Could you check a few things on this model? Use its own coordinates, in mm. Face numbers are marked on the shaded views. A direction names the side the tool comes from. Coordinates: 2 decimals unless noted, no trailing zeros. Loops run counter-clockwise (first coordinate to the right, second up) from the corner with the lowest first, then second, coordinate; pieces in that order, holes last.
1) Imagine slicing it at A-A on x = 0. Please give me the cut outline in (y, z).
2) If I drill on line 1 along Y through (x, z) = (0, 3.5); line 2 along Y through (x, z) = (2.25, 0.5); line 3 along X through (y, z) = (2.5, 4.75), over which ranges is the centre line in solid material (lowest first)?
3) For the marked faces 1 and 2, which set-ups out of +Z, -Z, +X, -X, +Y, -Y let a thin tool reach every point of the face, with its end or its side?
4) Will these pins go through, and if not, where does the flat tip stop? P1, Ø4, axis at y = -1, z = 6, coming from the +X side; P2, Ø3, axis at x = 1, z = 5.5, coming from the +Y side; P3, Ø1.5, axis at y = -2.5, z = -0.5, coming from the -X side.
5) Thinking about a two-plate mould opening in Y: for the marked faces 3, 4 and 5, which applies, released by +Y, released by -Y, zero draft, split by the parting line, or undercut?
6) Imagine slicing it at B-B on z = 6.75. Please give me the cut outline in (x, y), plus the area to 3 significant figures.
```python
from build123d import *

# Parameters (mm, degrees)
SKETCH2_R           = 4
SKETCH2_R_2         = 3.5
BOSS_EXTRUDE1_DEPTH = 8
SKETCH3_R           = 5
BOSS_EXTRUDE2_DEPTH = 2
BOSS_EXTRUDE2_TAPER = 30


with BuildPart() as part:
    # Sketch2 → Boss-Extrude1 (new body)
    with BuildSketch(Plane.XY):
        Circle(SKETCH2_R)
        Circle(SKETCH2_R_2, mode=Mode.SUBTRACT)
    extrude(amount=BOSS_EXTRUDE1_DEPTH)

    # Sketch3 → Boss-Extrude2 (add)
    with BuildSketch(Plane(origin=(0, 0, 0), x_dir=(-1, 0, 0), z_dir=(0, 0, -1))):
        Circle(SKETCH3_R)
    extrude(amount=BOSS_EXTRUDE2_DEPTH, taper=BOSS_EXTRUDE2_TAPER)


solid = part.part
```
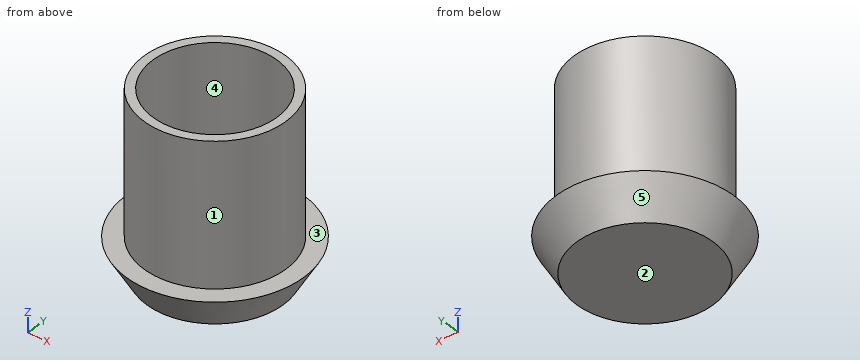
Filled in:
1. outline: (-5, 0) - (-3.85, -2) - (3.85, -2) - (5, 0) - (4, 0) - (4, 8) - (3.5, 8) - (3.5, 0) - (-3.5, 0) - (-3.5, 8) - (-4, 8) - (-4, 0) - close
2. line 1: y = -4 to -3.5, 3.5 to 4
2. line 2: y = -3.31 to -2.68, 2.68 to 3.31
2. line 3: x = -3.12 to -2.45, 2.45 to 3.12
3. face 1: +Z
3. face 2: -Z, +X, -X, +Y, -Y
4. P1: stops at x = 4
4. P2: stops at y = 4
4. P3: stops at x = -4.61
5. face 3: zero draft
5. face 4: undercut
5. face 5: split by the parting line
6. outline: circle Ø8 at (0, 0); hole circle Ø7 at (0, 0)
6. area: 11.8 mm2
